Verification items for the finished model (mm, model axes). Round coordinates to 2 decimals unless told otherwise and drop trailing zeros. Order: outer loops, then holes, each group sorted by start corner. A loop starts at its lowest first (then second) coordinate and runs counter-clockwise, first axis right, second up. Notation, with made-up numbers: M 46,-5 L 61,-5 A13 cw 61,8 Z; hole C -10,85 d11. An arc over 180 degrees is marked long. Return JSON: item names as keys, results as strings. Group by question number.
from build123d import *

# Parameters (mm, degrees)
ESQUISSE1_W                = 90
ESQUISSE1_H                = 189.15
BOSS_EXTRU_1_DEPTH         = 3
ESQUISSE2_W                = 10
ESQUISSE2_H                = 3
BOSS_EXTRU_2_DEPTH         = 3
R_P_TITION_LIN_AIRE1_COUNT = 5
R_P_TITION_LIN_AIRE1_PITCH = 20
ESQUISSE3_W                = 10
ESQUISSE3_H                = 3
BOSS_EXTRU_3_DEPTH         = 3
R_P_TITION_LIN_AIRE2_COUNT = 5
R_P_TITION_LIN_AIRE2_PITCH = 20
ESQUISSE4_W                = 3
ESQUISSE4_H                = 10
BOSS_EXTRU_4_DEPTH         = 3
R_P_TITION_LIN_AIRE3_COUNT = 9
R_P_TITION_LIN_AIRE3_PITCH = 20
ESQUISSE5_W                = 3
ESQUISSE5_H                = 10
BOSS_EXTRU_5_DEPTH         = 3
R_P_TITION_LIN_AIRE4_COUNT = 9
R_P_TITION_LIN_AIRE4_PITCH = 20


with BuildPart() as part:
    # Esquisse1 → Boss.-Extru.1 (new body)
    with BuildSketch(Plane.XY):
        with Locations((45, -94.575)):
            Rectangle(ESQUISSE1_W, ESQUISSE1_H)
    extrude(amount=BOSS_EXTRU_1_DEPTH)

    # Esquisse2 → Boss.-Extru.2 (add)
    with BuildSketch(Plane(origin=(0, 0, 0), x_dir=(1, 0, 0), z_dir=(0, 1, 0))):
        with Locations((5, -1.5)):
            Rectangle(ESQUISSE2_W, ESQUISSE2_H)
    boss_extru_2 = extrude(amount=BOSS_EXTRU_2_DEPTH)

    # Répétition linéaire1: Boss.-Extru.2 ×5
    with Locations(*[(i * R_P_TITION_LIN_AIRE1_PITCH, 0, 0) for i in range(1, R_P_TITION_LIN_AIRE1_COUNT)]):
        add(boss_extru_2)

    # Esquisse3 → Boss.-Extru.3 (add)
    with BuildSketch(Plane.XZ.offset(189.15)):
        with Locations((5, 1.5)):
            Rectangle(ESQUISSE3_W, ESQUISSE3_H)
    boss_extru_3 = extrude(amount=BOSS_EXTRU_3_DEPTH)

    # Répétition linéaire2: Boss.-Extru.3 ×5
    with Locations(*[(i * R_P_TITION_LIN_AIRE2_PITCH, 0, 0) for i in range(1, R_P_TITION_LIN_AIRE2_COUNT)]):
        add(boss_extru_3)

    # Esquisse4 → Boss.-Extru.4 (add)
    with BuildSketch(Plane.ZY):
        with Locations((1.5, -184.15)):
            Rectangle(ESQUISSE4_W, ESQUISSE4_H)
    boss_extru_4 = extrude(amount=BOSS_EXTRU_4_DEPTH)

    # Répétition linéaire3: Boss.-Extru.4 ×9
    with Locations(*[(0, i * R_P_TITION_LIN_AIRE3_PITCH, 0) for i in range(1, R_P_TITION_LIN_AIRE3_COUNT)]):
        add(boss_extru_4)

    # Esquisse5 → Boss.-Extru.5 (add)
    with BuildSketch(Plane(origin=(90, 0, 0), x_dir=(0, 0, -1), z_dir=(1, 0, 0))):
        with Locations((-1.5, -184.15)):
            Rectangle(ESQUISSE5_W, ESQUISSE5_H)
    boss_extru_5 = extrude(amount=BOSS_EXTRU_5_DEPTH)

    # Répétition linéaire4: Boss.-Extru.5 ×9
    with Locations(*[(0, i * R_P_TITION_LIN_AIRE4_PITCH, 0) for i in range(1, R_P_TITION_LIN_AIRE4_COUNT)]):
        add(boss_extru_5)


solid = part.part
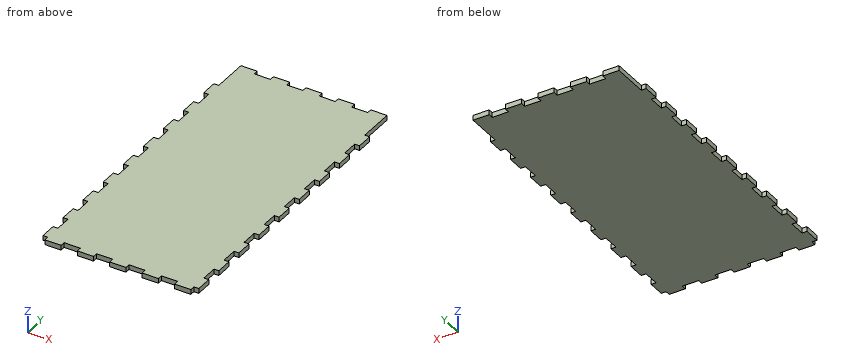
1. Cross-section at A-A (y = -171.5). Enter the section's corners in (x, z).
2. Thickness scan on line 1 along Y through (x, z) = (53, 0.6); line 2 along X through (y, z) = (-70.5, 1.45). Record the ranges inside material, lowest first. Write a range as from..to.
3. Go/stop test with flat-tipped pins: pin 1 (0.9 mm diameter, centred on y = -115.5, z = 1.5, fed in from -X); pin 2 (0.9 mm diameter, centred on y = -190.5, z = 1, fed in from +X); pin 3 (0.9 mm diameter, centred on x = 57.5, z = 1, fed in from -Y). Record where each tip stops, or that it passes through.
4. Cross-section at B-B (x = 34). Enter the section's corners in (y, z), plus the area to 3 significant figures.
Computed:
{
 "1": {"outline": "M 0,0 L 90,0 L 90,3 L 0,3 Z"},
 "2": {"line 1": "y = -189.15..0", "line 2": "x = 0..90"},
 "3": {"pin 1": "stops at x = 0", "pin 2": "stops at x = 90", "pin 3": "stops at y = -189.15"},
 "4": {"outline": "M -189.15,0 L 0,0 L 0,3 L -189.15,3 Z", "area": "567 mm²"}
}
